Part model, mm, in its own coordinate system. A direction names the side the tool comes from. Give positions to 0.01 mm unless a question says otherwise; leave off trailing zeros. Order: outer loops, then holes, each group sorted by start corner. A loop starts at its lowest first (then second) coordinate and runs counter-clockwise, first axis right, second up. Notation, with made-up numbers: M 22,34.25 L 52,34.25 A13 cw 52,49.25 Z; hole C 86,88 d11. An arc over 180 degrees is marked long. Return JSON: item names as keys, results as strings.
from build123d import *

# Parameters (mm, degrees)
F0_W     = 35
F0_H     = 25
F0_R     = 1.6
F0_W_2   = 20
F0_H_2   = 20
F1_DEPTH = 4.1
F2_W     = 35
F2_H     = 25
F2_R     = 3.15
F2_W_2   = 18
F2_H_2   = 18
F3_DEPTH = 14.1
F4_W     = 35
F4_H     = 25
F4_R     = 3.15
F4_W_2   = 14
F4_H_2   = 14
F5_DEPTH = 2
F6_W     = 18
F6_H     = 18
F7_DEPTH = 5


with BuildPart() as f1:
    # F0 (on Front) → F1 (new body)
    with BuildSketch(Plane.XZ):
        Rectangle(F0_W, F0_H)
        with Locations((-13, 0)):
            Circle(F0_R, mode=Mode.SUBTRACT)
        Rectangle(F0_W_2, F0_H_2, mode=Mode.SUBTRACT)
        with Locations((13, 0)):
            Circle(F0_R, mode=Mode.SUBTRACT)
    extrude(amount=F1_DEPTH)

    # F2 (on face) → F3 (join)
    with BuildSketch(Plane.XZ.offset(4.1)):
        Rectangle(F2_W, F2_H)
        with Locations((-13, 0)):
            Circle(F2_R, mode=Mode.SUBTRACT)
        Rectangle(F2_W_2, F2_H_2, mode=Mode.SUBTRACT)
        with Locations((13, 0)):
            Circle(F2_R, mode=Mode.SUBTRACT)
    extrude(amount=F3_DEPTH)

    # F4 (on face) → F5 (join)
    with BuildSketch(Plane.XZ.offset(18.2)):
        Rectangle(F4_W, F4_H)
        with Locations((-13, 0)):
            Circle(F4_R, mode=Mode.SUBTRACT)
        Rectangle(F4_W_2, F4_H_2, mode=Mode.SUBTRACT)
        with Locations((13, 0)):
            Circle(F4_R, mode=Mode.SUBTRACT)
    extrude(amount=F5_DEPTH)

    # F6 (on face) → F7 (cut)
    with BuildSketch(Plane(origin=(0, -4.1, 0), x_dir=(-1, 0, 0), z_dir=(0, 1, 0))):
        Rectangle(F6_W, F6_H)
    extrude(amount=-F7_DEPTH, mode=Mode.SUBTRACT)


solid = f1.part
Q1. Probe line 1 along X through (y, z) = (-8.5, 0); line 2 along X through (y, z) = (-18.25, 4.25); line 3 along Z through (x, y) = (-13, -9.75). List the from-to ranges inside material, lowest first.
Established:
{"line 1": "x = -17.5 to -16.15, -9.85 to -9, 9 to 9.85, 16.15 to 17.5", "line 2": "x = -17.5 to -7, 7 to 17.5", "line 3": "z = -12.5 to -3.15, 3.15 to 12.5"}
Q2. Band-saw the part on B-B (z = -4.5). Give the cut face in (x, y), then the cut area to 3 significant figures.
Established:
{"outline": "M -17.5,-20.2 L -7,-20.2 L -7,-18.2 L -9,-18.2 L -9,-4.1 L -10,-4.1 L -10,0 L -17.5,0 Z; M 7,-20.2 L 17.5,-20.2 L 17.5,0 L 10,0 L 10,-4.1 L 9,-4.1 L 9,-18.2 L 7,-18.2 Z", "area": "343 mm²"}
Q3. Band-saw the part on D-D (x = -13). Give the cut face in (y, z), then the cut area to 3 significant figures.
Established:
{"outline": "M -20.2,-12.5 L 0,-12.5 L 0,-1.6 L -4.1,-1.6 L -4.1,-3.15 L -20.2,-3.15 Z; M -20.2,3.15 L -4.1,3.15 L -4.1,1.6 L 0,1.6 L 0,12.5 L -20.2,12.5 Z", "area": "390 mm²"}
Q4. Pin check, flat tips, straight feed: pin 1 (5.5 mm diameter, centred on x = -13, z = 0, fed in from -Y); pin 2 (2 mm diameter, centred on x = -4.5, z = -9.5, fed in from +Y); pin 3 (6 mm diameter, centred on x = -3, z = -0.5, fed in from +Y). Stop position of each tip, or through.
Established:
{"pin 1": "stops at y = -4.1", "pin 2": "stops at y = 0", "pin 3": "passes through"}
Q5. Band-saw the part on A-A (x = -2). Give the cut face in (y, z), then the cut area to 3 significant figures.
Established:
{"outline": "M -20.2,-12.5 L 0,-12.5 L 0,-10 L -4.1,-10 L -4.1,-9 L -18.2,-9 L -18.2,-7 L -20.2,-7 Z; M -20.2,7 L -18.2,7 L -18.2,9 L -4.1,9 L -4.1,10 L 0,10 L 0,12.5 L -20.2,12.5 Z", "area": "141 mm²"}
Q6. 3-axis set-ups, long thin cutter, end or side, ignore diameter. For faces 4 (the flat face through (-9, -11, 0)), 5 (the flat face through (8, -20.2, 0)), 6 (the flat face through (7, -19, 0)), 7 (the cylindrical face through (-16.147, -12.037, 0.138)), 8 (the flat face through (0, 0, -11)): which of +Z, -Z, +X, -X, +Y, -Y reach the whole face in a straight line?
Established:
{"face 4": "+Y", "face 5": "+Z, -Z, +X, -X, -Y", "face 6": "+Y, -Y", "face 7": "-Y", "face 8": "+Z, -Z, +X, -X, +Y"}
Q7. Two-plate mould, pull along Z, no slides. Class faces 1 (the flat face through (-17.5, -10, 0)), 2 (the flat face through (0, -10, 12.5)), 3 (the cylindrical face through (-14.6, -2.02, 0.07)): +Z half, -Z half, draft (parallel to the pull), parting line (faces both ways), or undercut.
Established:
{"face 1": "draft", "face 2": "+Z half", "face 3": "undercut"}
Q8. Band-saw the part on C-C (y = -3.25). Give the cut face in (x, z), then the cut area to 3 significant figures.
Established:
{"outline": "M -17.5,-12.5 L 17.5,-12.5 L 17.5,12.5 L -17.5,12.5 Z; hole C -13,0 d3.2; hole M -10,-10 L 10,-10 L 10,10 L -10,10 Z; hole C 13,0 d3.2", "area": "459 mm²"}
